Verification items for the finished model (mm, model axes). A direction names the side the tool comes from. Round coordinates to 2 decimals unless told otherwise and drop trailing zeros. Write each loop counter-clockwise with the first axis right and the second up, starting at its lowest first coordinate (ties: lowest second). Pieces come first, ordered by that corner, then holes. Notation, with made-up numbers: (-23, -16.5) - (27, -16.5) arc R22 cw to (27, -10.5) - close; hole circle Ø3 at (-38, 5). An arc over 180 degrees is marked (long way). Answer as a JSON object with one key per item and string values.
```python
from build123d import *

# Parameters (mm, degrees)
EXTRUDE_1_DEPTH      = 55
CUT_EXTRUDE_START    = -5
SKETCH_2_R           = 18.75
SKETCH_2_R_2         = 14.75
CUT_EXTRUDE_1_DEPTH  = 59.016862823
EXTRUDE_3_REACH      = 65.017
EXTRUDE_3_END_RADIUS = 18.75
SKETCH_4_W           = 7
SKETCH_4_H           = 7
SKETCH_3_R           = 1.1
CUT_EXTRUDE_2_DEPTH  = 5
SKETCH_5_R           = 1.1
CUT_EXTRUDE_3_DEPTH  = 5
CUT_EXTRUDE_START_2  = -22
CUT_EXTRUDE_4_DEPTH  = 17
EXTRUDE_4_DEPTH      = 17
SKETCH_7_R           = 6.5
CUT_EXTRUDE_5_DEPTH  = 63.440972126
EXTRUDE_START        = -3
EXTRUDE_5_DEPTH      = 3
EXTRUDE_START_2      = 8
EXTRUDE_6_DEPTH      = 8
CUT_EXTRUDE_6_REACH  = 65.55
SKETCH_11_W          = 2
SKETCH_11_H          = 5


with BuildPart() as part:
    # ｽｹｯﾁ1 → ﾎﾞｽ - 押し出し1 (new body)
    with BuildSketch(Plane(origin=(0, 0, 0), x_dir=(1, 0, 0), z_dir=(0, 1, 0))):
        with BuildLine():
            Line((0, -21.75), (0, -14.75))
            ThreePointArc((0, -14.75), (-14.75, 0), (0, 14.75))
            Line((0, 14.75), (0, 21.75))
            ThreePointArc((0, 21.75), (-21.75, 0), (0, -21.75))
        make_face()
    extrude(amount=EXTRUDE_1_DEPTH)

    # ｽｹｯﾁ2 → ｶｯﾄ - 押し出し1 (cut, through all)
    with BuildSketch(Plane(origin=(0, 55, 0), x_dir=(1, 0, 0), z_dir=(0, 1, 0)).offset(CUT_EXTRUDE_START)):
        Circle(SKETCH_2_R)
        Circle(SKETCH_2_R_2, mode=Mode.SUBTRACT)
    extrude(amount=-CUT_EXTRUDE_1_DEPTH, mode=Mode.SUBTRACT)

    # ﾎﾞｽ - 押し出し3: up to this cylinder (the profile starts inside it)
    extrude_3_end = Plane(origin=(0, 25, 0), z_dir=(0, 1, 0)) * Cylinder(EXTRUDE_3_END_RADIUS, 193.534, mode=Mode.PRIVATE)
    # ｽｹｯﾁ4 → ﾎﾞｽ - 押し出し3 (add, up to the surface)
    with BuildSketch(Plane(origin=(0, 0, 0), x_dir=(0, 0, -1), z_dir=(1, 0, 0)), mode=Mode.PRIVATE) as extrude_3_sk1:
        with Locations((-18.25, 37.5)):
            Rectangle(SKETCH_4_W, SKETCH_4_H)
    extrude_3_tool1 = extrude(extrude_3_sk1.sketch, amount=-EXTRUDE_3_REACH, mode=Mode.PRIVATE) & extrude_3_end
    add(extrude_3_tool1.solids().sort_by_distance((0, 37.5, 18.25))[0])
    # ｽｹｯﾁ4 → ﾎﾞｽ - 押し出し3 (add, up to the surface)
    with BuildSketch(Plane(origin=(0, 0, 0), x_dir=(0, 0, -1), z_dir=(1, 0, 0)), mode=Mode.PRIVATE) as extrude_3_sk2:
        with Locations((-18.25, 12.5)):
            Rectangle(SKETCH_4_W, SKETCH_4_H)
    extrude_3_tool2 = extrude(extrude_3_sk2.sketch, amount=-EXTRUDE_3_REACH, mode=Mode.PRIVATE) & extrude_3_end
    add(extrude_3_tool2.solids().sort_by_distance((0, 12.5, 18.25))[0])
    # ｽｹｯﾁ4 → ﾎﾞｽ - 押し出し3 (add, up to the surface)
    with BuildSketch(Plane(origin=(0, 0, 0), x_dir=(0, 0, -1), z_dir=(1, 0, 0)), mode=Mode.PRIVATE) as extrude_3_sk3:
        with Locations((18.25, 12.5)):
            Rectangle(SKETCH_4_W, SKETCH_4_H)
    extrude_3_tool3 = extrude(extrude_3_sk3.sketch, amount=-EXTRUDE_3_REACH, mode=Mode.PRIVATE) & extrude_3_end
    add(extrude_3_tool3.solids().sort_by_distance((0, 12.5, -18.25))[0])
    # ｽｹｯﾁ4 → ﾎﾞｽ - 押し出し3 (add, up to the surface)
    with BuildSketch(Plane(origin=(0, 0, 0), x_dir=(0, 0, -1), z_dir=(1, 0, 0)), mode=Mode.PRIVATE) as extrude_3_sk4:
        with Locations((18.25, 37.5)):
            Rectangle(SKETCH_4_W, SKETCH_4_H)
    extrude_3_tool4 = extrude(extrude_3_sk4.sketch, amount=-EXTRUDE_3_REACH, mode=Mode.PRIVATE) & extrude_3_end
    add(extrude_3_tool4.solids().sort_by_distance((0, 37.5, -18.25))[0])

    # ｽｹｯﾁ3 → ｶｯﾄ - 押し出し2 (cut)
    with BuildSketch(Plane(origin=(0, 0, 0), x_dir=(0, 0, -1), z_dir=(1, 0, 0))):
        with Locations((-18.25, 37.5)):
            Circle(SKETCH_3_R)
        with Locations(Location((18.25, 37.5, 0), (0, 0, 180))):
            Circle(SKETCH_3_R)
        with Locations((18.25, 12.5)):
            Circle(SKETCH_3_R)
        with Locations(Location((-18.25, 12.5, 0), (0, 0, 180))):
            Circle(SKETCH_3_R)
    extrude(amount=-CUT_EXTRUDE_2_DEPTH, mode=Mode.SUBTRACT)

    # ｽｹｯﾁ5 → ｶｯﾄ - 押し出し3 (cut)
    with BuildSketch(Plane(origin=(0, 55, 0), x_dir=(1, 0, 0), z_dir=(0, 1, 0))):
        with Locations(Location((-12.904698757, -12.904698757, 0), (0, 0, 270))):
            Circle(SKETCH_5_R)
        with Locations(Location((-12.904698757, 12.904698757, 0), (0, 0, 270))):
            Circle(SKETCH_5_R)
    extrude(amount=-CUT_EXTRUDE_3_DEPTH, mode=Mode.SUBTRACT)

    # ｽｹｯﾁ6 → ｶｯﾄ - 押し出し4 (cut)
    with BuildSketch(Plane(origin=(0, 55, 0), x_dir=(1, 0, 0), z_dir=(0, 1, 0)).offset(CUT_EXTRUDE_START_2)):
        with BuildLine():
            Line((-20.020302196, 8.5), (-20.020302196, -8.5))
            ThreePointArc((-20.020302196, -8.5), (-21.75, 0), (-20.020302196, 8.5))
        make_face()
    extrude(amount=CUT_EXTRUDE_4_DEPTH, mode=Mode.SUBTRACT)

    # ｽｹｯﾁ8 → ﾎﾞｽ - 押し出し4 (add)
    with BuildSketch(Plane.XZ.offset(-50)):
        with BuildLine():
            Line((-16.712644913, 8.5), (-16.712644913, -8.5))
            ThreePointArc((-16.712644913, -8.5), (-18.75, 0), (-16.712644913, 8.5))
        make_face()
    extrude(amount=EXTRUDE_4_DEPTH)

    # ｽｹｯﾁ7 → ｶｯﾄ - 押し出し5 (cut, through all)
    with BuildSketch(Plane.ZY.offset(20.020302196)):
        with Locations((0, 41.5)):
            Circle(SKETCH_7_R)
    extrude(amount=-CUT_EXTRUDE_5_DEPTH, mode=Mode.SUBTRACT)

    # ｽｹｯﾁ9 → ﾎﾞｽ - 押し出し5 (add)
    with BuildSketch(Plane.XZ.offset(EXTRUDE_START)):
        with BuildLine():
            Line((0, 18.75), (0, 3.95))
            ThreePointArc((0, 3.95), (-3.95, 0), (0, -3.95))
            Line((0, -3.95), (0, -18.75))
            ThreePointArc((0, -18.75), (-18.75, 0), (0, 18.75))
        make_face()
    extrude(amount=EXTRUDE_5_DEPTH)

    # ｽｹｯﾁ10 → ﾎﾞｽ - 押し出し6 (add)
    with BuildSketch(Plane(origin=(0, 3, 0), x_dir=(1, 0, 0), z_dir=(0, 1, 0)).offset(EXTRUDE_START_2)):
        with BuildLine():
            Line((-3.654107278, -1.5), (-11.654107278, -1.5))
            Line((-11.654107278, -1.5), (-11.654107278, 1.5))
            Line((-11.654107278, 1.5), (-3.654107278, 1.5))
            ThreePointArc((-3.654107278, 1.5), (-3.95, 0), (-3.654107278, -1.5))
        make_face()
    extrude(amount=-EXTRUDE_6_DEPTH)

    # ｽｹｯﾁ11 → ｶｯﾄ - 押し出し6 (cut, up to next)
    with BuildSketch(Plane.XY.offset(1.5), mode=Mode.PRIVATE) as cut_extrude_6_sk1:
        with Locations((-7.654107278, 5.5)):
            Rectangle(SKETCH_11_W, SKETCH_11_H)
    cut_extrude_6_tool1 = extrude(cut_extrude_6_sk1.sketch, amount=-CUT_EXTRUDE_6_REACH, mode=Mode.PRIVATE) & part.part
    add(cut_extrude_6_tool1.solids().sort_by_distance((-7.654107, 5.5, 1.5))[0], mode=Mode.SUBTRACT)


solid = part.part
```
Q1. Material ranges on line 1 along Y through (x, z) = (-3.45, 18.25); line 2 along Y through (x, z) = (-3, 15); line 3 along Y through (x, z) = (-13.5, -8), recorded low to high. Write a range as [from, to].
Geometry check:
{"line 1": "y = [0, 3], [9, 11.4], [13.6, 16], [34, 36.4], [38.6, 41], [50, 55]", "line 2": "y = [0, 3], [9, 16], [34, 41], [50, 55]", "line 3": "y = [0, 3], [50, 55]"}
Q2. Section check B-B, the plane y = 12.5. Record the cut outline in (x, z), then the cut area to 3 significant figures.
Geometry check:
{"outline": "(-11.58, -14.75) arc R18.75 cw to (-11.58, 14.75) - (0, 14.75) - (0, 17.15) - (-5, 17.15) - (-5, 19.35) - (0, 19.35) - (0, 21.75) arc R21.75 ccw to (0, -21.75) - (0, -19.35) - (-5, -19.35) - (-5, -17.15) - (0, -17.15) - (0, -14.75) - close", "area": "232 mm2"}
Q3. Gauge pin test, flat ends, axial feed: P1, Ø6, axis at x = -5, z = 0.5, coming from the -Y side; P2, Ø3, axis at x = -15, y = 12, coming from the +Z side; P3, Ø4, axis at x = -6.5, y = 6, coming from the -Z side; P4, Ø7.5, axis at x = -4, y = 37.5, coming from the +Z side. Record the tip position at first contact, or that the pin passes through.
Geometry check:
{"P1": "stops at y = 0", "P2": "stops at z = 17.05", "P3": "stops at z = -21.28", "P4": "stops at z = 21.75"}
Q4. Section check A-A, the plane z = 0. Record the cut outline in (x, y).
Geometry check:
{"outline": "(-21.75, 0) - (-3.95, 0) - (-3.95, 11) - (-11.65, 11) - (-11.65, 3) - (-18.75, 3) - (-18.75, 33) - (-16.71, 33) - (-16.71, 35) - (-20.02, 35) - (-20.02, 33) - (-21.75, 33) - close; (-21.75, 50) - (-20.02, 50) - (-20.02, 48) - (-16.71, 48) - (-16.71, 50) - (-14.75, 50) - (-14.75, 55) - (-21.75, 55) - close; hole (-8.65, 3) - (-6.65, 3) - (-6.65, 8) - (-8.65, 8) - close"}
Q5. Set-up check for faces 1 (the flat face through (-4, 9, -16)), 2 (the flat face through (-20.02, 36, 4)), 3 (the flat face through (-8, 8, 0)), 4 (the flat face through (-13.4, 50, -13.4)): record each of +Z, -Z, +X, -X, +Y, -Y from which the full face is reachable in a straight line by a thin tool's end or side.
Geometry check:
{"face 1": "+X", "face 2": "+Z, -Z, -X", "face 3": "none", "face 4": "+Y"}
Q6. Release check for a two-part mould opening along X. For faces 5 (the cylindrical face through (-13, 53, 14)), 6 (the flat face through (-6, 12, 14.75)), 7 (the flat face through (-16.713, 47, -4)) record: released by +X, released by -X, zero draft, split by the parting line, or undercut.
Geometry check:
{"face 5": "undercut", "face 6": "zero draft", "face 7": "released by +X"}
Q7. Section check D-D, the plane x = -1.25. State how many separate pieces and enclosed holes the cut face has, then the cut area to 3 significant figures.
Geometry check:
{"separate pieces": "2", "enclosed holes": "4", "area": "556 mm2"}
Q8. Section check C-C, the plane y = 37.5. Record the cut outline in (x, z).
Geometry check:
{"outline": "(-20.02, -8.5) arc R21.75 ccw to (0, -21.75) - (0, -19.35) - (-5, -19.35) - (-5, -17.15) - (0, -17.15) - (0, -14.75) - (-11.58, -14.75) arc R18.75 cw to (-16.71, -8.5) - (-16.71, -5.12) - (-20.02, -5.12) - close; (-20.02, 5.12) - (-16.71, 5.12) - (-16.71, 8.5) arc R18.75 cw to (-11.58, 14.75) - (0, 14.75) - (0, 17.15) - (-5, 17.15) - (-5, 19.35) - (0, 19.35) - (0, 21.75) arc R21.75 ccw to (-20.02, 8.5) - close"}
